```python
from build123d import *

# Parameters (mm, degrees)
SKETCH1_R                  = 9.75
BOSS_EXTRUDE1_DEPTH        = 60
M2_TAPPED_HOLE1_AT_2_COUNT = 2
M2_TAPPED_HOLE1_AT_2_PITCH = 6.122934918
M2_TAPPED_HOLE1_AT_3_COUNT = 2
M2_TAPPED_HOLE1_AT_3_PITCH = 11.313708499
M2_TAPPED_HOLE1_AT_4_COUNT = 2
M2_TAPPED_HOLE1_AT_4_PITCH = 14.78207252
M2_TAPPED_HOLE1_AT_5_COUNT = 2
M2_TAPPED_HOLE1_AT_5_PITCH = 16
M2_TAPPED_HOLE1_AT_6_COUNT = 2
M2_TAPPED_HOLE1_AT_6_PITCH = 14.78207252
M2_TAPPED_HOLE1_AT_7_COUNT = 2
M2_TAPPED_HOLE1_AT_7_PITCH = 11.313708499
M2_TAPPED_HOLE1_AT_8_COUNT = 2
M2_TAPPED_HOLE1_AT_8_PITCH = 6.122934918


with BuildPart() as part:
    # Sketch1 → Boss-Extrude1 (new body)
    with BuildSketch(Plane(origin=(0, 0, 0), x_dir=(0, 0, -1), z_dir=(1, 0, 0))):
        Circle(SKETCH1_R)
    extrude(amount=BOSS_EXTRUDE1_DEPTH)

    # Sketch4 → M2 Tapped Hole1 (revolve, cut)
    with BuildSketch(Plane(origin=(60, 8, 0), x_dir=(0, 0, -1), z_dir=(0, 1, 0))):
        Polygon((0, 0), (0, 5.680688495), (0.8, 5.2), (0.8, 0), align=None)
    m2_tapped_hole1 = revolve(axis=Axis((66.35, 8, 0), (-1, 0, 0)), mode=Mode.SUBTRACT)

    # M2 Tapped Hole1 at 2: M2 Tapped Hole1 ×2
    with Locations(*[Vector(0, -0.3826834323650503, -0.9238795325113031) * (i * M2_TAPPED_HOLE1_AT_2_PITCH) for i in range(1, M2_TAPPED_HOLE1_AT_2_COUNT)]):
        add(m2_tapped_hole1, mode=Mode.SUBTRACT)

    # M2 Tapped Hole1 at 3: M2 Tapped Hole1 ×2
    with Locations(*[Vector(0, -0.7071067811865174, -0.7071067811865777) * (i * M2_TAPPED_HOLE1_AT_3_PITCH) for i in range(1, M2_TAPPED_HOLE1_AT_3_COUNT)]):
        add(m2_tapped_hole1, mode=Mode.SUBTRACT)

    # M2 Tapped Hole1 at 4: M2 Tapped Hole1 ×2
    with Locations(*[Vector(0, -0.9238795325112705, -0.38268343236512903) * (i * M2_TAPPED_HOLE1_AT_4_PITCH) for i in range(1, M2_TAPPED_HOLE1_AT_4_COUNT)]):
        add(m2_tapped_hole1, mode=Mode.SUBTRACT)

    # M2 Tapped Hole1 at 5: M2 Tapped Hole1 ×2
    with Locations(*[(0, -i * M2_TAPPED_HOLE1_AT_5_PITCH, 0) for i in range(1, M2_TAPPED_HOLE1_AT_5_COUNT)]):
        add(m2_tapped_hole1, mode=Mode.SUBTRACT)

    # M2 Tapped Hole1 at 6: M2 Tapped Hole1 ×2
    with Locations(*[Vector(0, -0.9238795325113031, 0.3826834323650506) * (i * M2_TAPPED_HOLE1_AT_6_PITCH) for i in range(1, M2_TAPPED_HOLE1_AT_6_COUNT)]):
        add(m2_tapped_hole1, mode=Mode.SUBTRACT)

    # M2 Tapped Hole1 at 7: M2 Tapped Hole1 ×2
    with Locations(*[Vector(0, -0.7071067811865777, 0.7071067811865174) * (i * M2_TAPPED_HOLE1_AT_7_PITCH) for i in range(1, M2_TAPPED_HOLE1_AT_7_COUNT)]):
        add(m2_tapped_hole1, mode=Mode.SUBTRACT)

    # M2 Tapped Hole1 at 8: M2 Tapped Hole1 ×2
    with Locations(*[Vector(0, -0.3826834323651289, 0.9238795325112706) * (i * M2_TAPPED_HOLE1_AT_8_PITCH) for i in range(1, M2_TAPPED_HOLE1_AT_8_COUNT)]):
        add(m2_tapped_hole1, mode=Mode.SUBTRACT)

    # Mirror1: M2 Tapped Hole1 across plane
    add(m2_tapped_hole1.mirror(Plane(origin=(30, 0, 0), x_dir=(0, 0, 1), z_dir=(1, 0, 0))), mode=Mode.SUBTRACT)

    # Mirror1 copy 1 sketch → Mirror1 copy 1 (revolve, cut)
    with BuildSketch(Plane(origin=(0, 5.656854249, -5.656854249), x_dir=(0, 0, -1), z_dir=(0, 1, 0))):
        Polygon((0, 0), (0, -5.680688495), (0.8, -5.2), (0.8, 0), align=None)
    revolve(axis=Axis((-6.35, 5.656854249, -5.656854249), (-1, 0, 0)), mode=Mode.SUBTRACT)

    # Mirror1 copy 2 sketch → Mirror1 copy 2 (revolve, cut)
    with BuildSketch(Plane(origin=(0, 0, -8), x_dir=(0, 0, -1), z_dir=(0, 1, 0))):
        Polygon((0, 0), (0, -5.680688495), (0.8, -5.2), (0.8, 0), align=None)
    revolve(axis=Axis((-6.35, 0, -8), (-1, 0, 0)), mode=Mode.SUBTRACT)

    # Mirror1 copy 3 sketch → Mirror1 copy 3 (revolve, cut)
    with BuildSketch(Plane(origin=(0, -5.656854249, -5.656854249), x_dir=(0, 0, -1), z_dir=(0, 1, 0))):
        Polygon((0, 0), (0, -5.680688495), (0.8, -5.2), (0.8, 0), align=None)
    revolve(axis=Axis((-6.35, -5.656854249, -5.656854249), (-1, 0, 0)), mode=Mode.SUBTRACT)

    # Mirror1 copy 4 sketch → Mirror1 copy 4 (revolve, cut)
    with BuildSketch(Plane(origin=(0, -8, 0), x_dir=(0, 0, -1), z_dir=(0, 1, 0))):
        Polygon((0, 0), (0, -5.680688495), (0.8, -5.2), (0.8, 0), align=None)
    revolve(axis=Axis((-6.35, -8, 0), (-1, 0, 0)), mode=Mode.SUBTRACT)

    # Mirror1 copy 5 sketch → Mirror1 copy 5 (revolve, cut)
    with BuildSketch(Plane(origin=(0, -5.656854249, 5.656854249), x_dir=(0, 0, -1), z_dir=(0, 1, 0))):
        Polygon((0, 0), (0, -5.680688495), (0.8, -5.2), (0.8, 0), align=None)
    revolve(axis=Axis((-6.35, -5.656854249, 5.656854249), (-1, 0, 0)), mode=Mode.SUBTRACT)

    # Mirror1 copy 6 sketch → Mirror1 copy 6 (revolve, cut)
    with BuildSketch(Plane(origin=(0, 0, 8), x_dir=(0, 0, -1), z_dir=(0, 1, 0))):
        Polygon((0, 0), (0, -5.680688495), (0.8, -5.2), (0.8, 0), align=None)
    revolve(axis=Axis((-6.35, 0, 8), (-1, 0, 0)), mode=Mode.SUBTRACT)

    # Mirror1 copy 7 sketch → Mirror1 copy 7 (revolve, cut)
    with BuildSketch(Plane(origin=(0, 5.656854249, 5.656854249), x_dir=(0, 0, -1), z_dir=(0, 1, 0))):
        Polygon((0, 0), (0, -5.680688495), (0.8, -5.2), (0.8, 0), align=None)
    revolve(axis=Axis((-6.35, 5.656854249, 5.656854249), (-1, 0, 0)), mode=Mode.SUBTRACT)


solid = part.part
```
Model file for the job. Use its own axes, mm. A direction names the side the tool comes from. Give positions to 0.01 mm unless a question says otherwise; leave off trailing zeros. Loops run counter-clockwise (first coordinate to the right, second up) from the corner with the lowest first, then second, coordinate; pieces in that order, holes last. Notation, with made-up numbers: (35, 86.25) -> (88, 86.25) arc R22 cw to (88, 108.25) -> close; hole circle Ø4 at (35.5, -12). An arc over 180 degrees is marked (long way). Use CSV: the item, a comma, the result in double quotes. Start each with the question number.
1) Wall check: line 1 (Y direction, x = 57.7, z = 0); line 2 (Z direction, x = 3.85, y = -8); line 3 (X direction, y = 0, z = -8). Give the ranges that are in metal, low to high.
2) Slice it at A-A on x = 43.5. Give the cut face in (y, z), plus the area to 3 significant figures.
3) Tool access for faces 1 (the cylindrical face through (57.44, -5.9, -6.42)), 2 (the cylindrical face through (2.56, -5.17, 6.29)): list every direction of +Z, -Z, +X, -X, +Y, -Y with a clear straight run to the whole face (end or side of a thin tool).
4) Mould opens along Z. For faces 3 (the flat face through (0, 0, 0)), 4 (the conical face through (54.403, -5.699, -5.789)) say: released by +Z, released by -Z, zero draft, split by the parting line, or undercut.
5) Flat gauge pins, fed straight in: pin 1 Ø1 at (y, z) = (0, -8) entering from -X; pin 2 Ø8 at (x, z) = (6.5, 6) entering from -Y; pin 3 Ø1.3 at (y, z) = (5.66, -5.66) entering from +X. Where does each tip first touch, or does it go through?
6) Slice it at B-B on z = -4.25. Give the cut face in (x, y), plus the area to 3 significant figures.
Computed values:
1,line 1,"y = -9.75 to -8.8, -7.2 to 7.2, 8.8 to 9.75"
1,line 2,"z = -5.57 to -0.8, 0.8 to 5.57"
1,line 3,"x = 5.68 to 54.32"
2,outline,"circle Ø19.5 at (0, 0)"
2,area,"299 mm^2"
3,face 1,"+X"
3,face 2,"-X"
4,face 3,"zero draft"
4,face 4,"undercut"
5,pin 1,"stops at x = 5.38"
5,pin 2,"stops at y = -9.54"
5,pin 3,"stops at x = 54.71"
6,outline,"(0, -8.77) -> (60, -8.77) -> (60, 8.77) -> (0, 8.77) -> close"
6,area,"1,050 mm^2"
